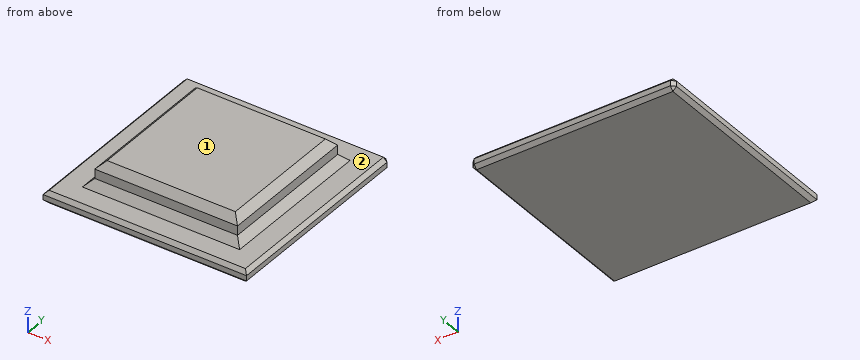
```python
from build123d import *

# Parameters (mm, degrees)
F0_W     = 142.24
F0_H     = 142.24
F1_DEPTH = 8.763
F2_W     = 99.7141572639
F2_H     = 99.7141572639
F3_DEPTH = 25.4
F4_SIZE  = 2.54
F5_SIZE  = 5.08


with BuildPart() as f1:
    # F0 (on Top) → F1 (new body)
    with BuildSketch(Plane.XY):
        Rectangle(F0_W, F0_H)
    extrude(amount=F1_DEPTH)

    # F2 (on Top) → F3 (join)
    with BuildSketch(Plane.XY):
        Rectangle(F2_W, F2_H)
    extrude(amount=F3_DEPTH)

    # F4
    f4_edges = [f1.edges().sort_by_distance(p)[0] for p in [
        (71.12, 71.12, 4.3815),
        (-71.12, 71.12, 4.3815),
        (0, 71.12, 0),
        (0, 71.12, 8.763),
        (71.12, 0, 8.763),
        (71.12, 0, 0),
        (0, -71.12, 8.763),
        (0, -71.12, 0),
        (-71.12, 0, 8.763),
        (-71.12, 0, 0),
    ]]
    chamfer(f4_edges, length=F4_SIZE)

    # F5
    f5_edges = [f1.edges().sort_by_distance(p)[0] for p in [
        (-49.857079, 0, 25.4),
        (0, 49.857079, 25.4),
        (0, -49.857079, 25.4),
        (49.857079, 0, 25.4),
        (-49.857079, 0, 8.763),
        (0, 49.857079, 8.763),
        (49.857079, 0, 8.763),
        (0, -49.857079, 8.763),
    ]]
    chamfer(f5_edges, length=F5_SIZE)


solid = f1.part
```
Can you work these out from the model? Positions are in its coordinate system, mm. Face numbers are marked on the shaded views. A direction names the side the tool comes from. Round coordinates to 2 decimals unless told otherwise and drop trailing zeros. Loops run counter-clockwise (first coordinate to the right, second up) from the corner with the lowest first, then second, coordinate; pieces in that order, holes last. Notation, with made-up numbers: (28.5, -36.75) -> (53.5, -36.75) arc R9 ccw to (53.5, -22.75) -> close; hole circle Ø3 at (76.5, 52.5). An arc over 180 degrees is marked (long way). Answer in a Markdown table with one row per item.
Item 1: Suppose I cut it at B-B, the plane y = -27. List the corners of the cut face in (x, z) for me.
Answer block:
| item | result |
|---|---|
| outline | (-71.12, 2.54) -> (-68.58, 0) -> (68.58, 0) -> (71.12, 2.54) -> (71.12, 6.22) -> (68.58, 8.76) -> (54.94, 8.76) -> (49.86, 13.84) -> (49.86, 20.32) -> (44.78, 25.4) -> (-44.78, 25.4) -> (-49.86, 20.32) -> (-49.86, 13.84) -> (-54.94, 8.76) -> (-68.58, 8.76) -> (-71.12, 6.22) -> close |
Item 2: Suppose I cut it at C-C, the plane z = 16.5. List the corners of the cut face in (x, y) for me, plus the area to 3 significant figures.
Answer block:
| item | result |
|---|---|
| outline | (-49.86, -49.86) -> (49.86, -49.86) -> (49.86, 49.86) -> (-49.86, 49.86) -> close |
| area | 9,940 mm² |
Item 3: Suppose I cut it at A-A, the plane x = 58. List the corners of the cut face in (y, z) for me, plus the area to 3 significant figures.
Answer block:
| item | result |
|---|---|
| outline | (-71.12, 2.54) -> (-68.58, 0) -> (68.58, 0) -> (71.12, 2.54) -> (71.12, 6.22) -> (68.58, 8.76) -> (-68.58, 8.76) -> (-71.12, 6.22) -> close |
| area | 1,230 mm² |
Item 4: Will these pins go through, and if not, where does the flat tip stop? P1, Ø2, axis at x = -10, z = 16.5, coming from the -Y side; P2, Ø7, axis at y = -14.5, z = 18.5, coming from the +X side; P3, Ø5, axis at x = 16.5, z = 13.5, coming from the +Y side.
Answer block:
| item | result |
|---|---|
| P1 | y = -49.86 |
| P2 | x = 49.86 |
| P3 | y = 52.7 |
Item 5: If I drill on probe 1 along Y at (x, z) = (-18, 2.5); probe 2 along Y at (x, z) = (23, 14); probe 3 along Z at (x, y) = (-60, 45.5), over which ranges is the centre line in solid material (lowest first)?
Answer block:
| item | result |
|---|---|
| probe 1 | -71.08 to 71.08 |
| probe 2 | -49.86 to 49.86 |
| probe 3 | 0 to 8.76 |
Item 6: On a 3-axis mill with a long thin cutter (end or side, diameter ignored), from which of +Z, -Z, +X, -X, +Y, -Y can I reach the whole of each face in a straight line? I mean the marked faces 1 and 2. Say none if no direction works.
Answer block:
| item | result |
|---|---|
| face 1 | +Z, +X, -X, +Y, -Y |
| face 2 | +Z |
